Geometry: final body of the model. Coordinates: model frame, mm. Round coordinates to 2 decimals unless told otherwise and drop trailing zeros. Loops run counter-clockwise (first coordinate to the right, second up) from the corner with the lowest first, then second, coordinate; pieces in that order, holes last. Notation, with made-up numbers: (3.5, 71) - (40.5, 71) arc R23 ccw to (40.5, 82) - close; hole circle Ø4 at (75.5, -20). An arc over 180 degrees is marked (long way). Return JSON: item names as keys, results as strings. Group by question number.
1. Section D-D on z = 54. Return loops of the section in (x, y), and give its area (3 significant figures).
2. Section B-B on x = 0.4. Return loops of the section in (y, z) (3 decimals), and give its area (3 significant figures).
3. Material intervals for probe 1 along Y at (x, z) = (-0.2, 0); probe 2 along Z at (x, y) = (-0.05, -3); probe 3 along Y at (x, z) = (-0.15, 50.5), sorted ascending.
4. Section A-A on y = 0. Return loops of the section in (x, z).
5. First-contact query: pin 1 Ø4 at (y, z) = (0, 0) entering from +X. Flat tip, straight axial feed; report the tip coordinate or a pass-through.
6. Section C-C on z = -1. Return loops of the section in (x, y), and give its area (3 significant figures).
from build123d import *

# Parameters (mm, degrees)
SKETCH1_R           = 3.2639
BOSS_EXTRUDE1_DEPTH = 0.79375
BOSS_EXTRUDE2_DEPTH = 1.5875


with BuildPart() as part:
    # Sketch1 → Boss-Extrude1 (new, symmetric)
    with BuildSketch(Plane(origin=(0, 0, 0), x_dir=(0, 0, -1), z_dir=(1, 0, 0))):
        with BuildLine():
            Line((-76.2, 9.525), (-76.2, -9.525))
            Line((-76.2, -9.525), (0.260118416, -6.433643728))
            ThreePointArc((0.260118416, -6.433643728), (6.4389, 0), (0.260118416, 6.433643728))
            Line((0.260118416, 6.433643728), (-76.2, 9.525))
        make_face()
        Circle(SKETCH1_R, mode=Mode.SUBTRACT)
    extrude(amount=BOSS_EXTRUDE1_DEPTH, both=True)

    # Sketch2 → Boss-Extrude2 (add)
    with BuildSketch(Plane.ZY.offset(0.79375)):
        Polygon((61.8850913, -8.946234446), (49.1954587, -8.433180371), (49.131326941, -10.019384446), (61.82095954, -10.532438521), align=None)
        Polygon((49.131326941, 10.019384446), (49.1954587, 8.433180371), (61.8850913, 8.946234446), (61.82095954, 10.532438521), align=None)
    extrude(amount=-BOSS_EXTRUDE2_DEPTH)


solid = part.part
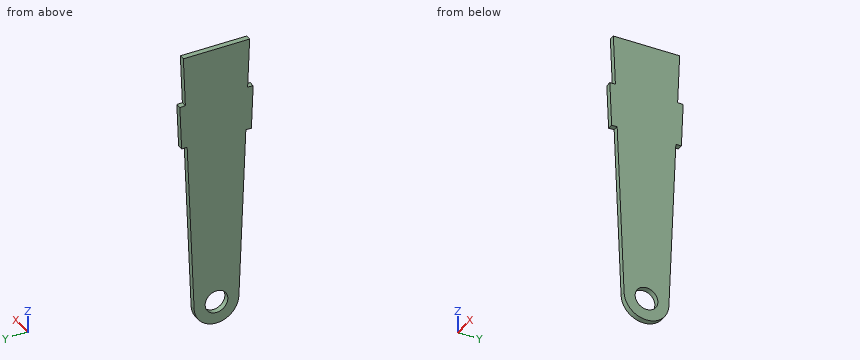
Taken from the geometry:
{
 "1": {"outline": "(-0.79, -10.22) - (0.79, -10.22) - (0.79, 10.22) - (-0.79, 10.22) - close", "area": "32.4 mm2"},
 "2": {"outline": "(-10.532, 61.821) - (-10.019, 49.131) - (-8.433, 49.195) - (-6.434, -0.26) arc R6.439 ccw to (6.434, -0.26) - (8.433, 49.195) - (10.019, 49.131) - (10.532, 61.821) - (8.946, 61.885) - (9.525, 76.2) - (-9.525, 76.2) - (-8.946, 61.885) - close; hole circle Ø6.528 at (0, 0)", "area": "1,290 mm2"},
 "3": {"probe 1": "-6.44 to -3.26, 3.26 to 6.44", "probe 2": "-5.7 to -1.29, 1.29 to 76.2", "probe 3": "-10.07 to 10.07"},
 "4": {"outline": "(-0.79, -6.44) - (0.79, -6.44) - (0.79, -3.26) - (-0.79, -3.26) - close; (-0.79, 3.26) - (0.79, 3.26) - (0.79, 76.2) - (-0.79, 76.2) - close"},
 "5": {"pin 1": "through"},
 "6": {"outline": "(-0.79, -6.36) - (0.79, -6.36) - (0.79, -3.11) - (-0.79, -3.11) - close; (-0.79, 3.11) - (0.79, 3.11) - (0.79, 6.36) - (-0.79, 6.36) - close", "area": "10.3 mm2"}
}
